from build123d import *

# Parameters (mm, degrees)
F0_R     = 35
F0_R_2   = 19
F0_R_3   = 1.5
F0_R_4   = 6.5
F0_R_5   = 3.5
F1_DEPTH = 20
F2_DEPTH = 7
F3_DEPTH = 13.75


with BuildPart() as f1:
    # F0 (on Top) → F1 (new body)
    with BuildSketch(Plane.XY):
        Circle(F0_R)
        with Locations((-7, 0)):
            Circle(F0_R_2, mode=Mode.SUBTRACT)
        with Locations((-7, 0)):
            Circle(F0_R_2)
        with Locations((-20.1270902899, -8.2419354839)):
            Circle(F0_R_3, mode=Mode.SUBTRACT)
        with Locations((-7, -15.5)):
            Circle(F0_R_3, mode=Mode.SUBTRACT)
        with Locations((6.1270902899, -8.2419354839)):
            Circle(F0_R_3, mode=Mode.SUBTRACT)
        with Locations((-20.1270902899, 8.2419354839)):
            Circle(F0_R_3, mode=Mode.SUBTRACT)
        with Locations((-7, 15.5)):
            Circle(F0_R_3, mode=Mode.SUBTRACT)
        Circle(F0_R_4, mode=Mode.SUBTRACT)
        with Locations((6.1270902899, 8.2419354839)):
            Circle(F0_R_3, mode=Mode.SUBTRACT)
        Circle(F0_R_4)
        Circle(F0_R_5, mode=Mode.SUBTRACT)
    extrude(amount=F1_DEPTH)

    # F0 (on Top) → F2 (cut)
    with BuildSketch(Plane.XY):
        with Locations((-7, 0)):
            Circle(F0_R_2)
        with Locations((-20.1270902899, -8.2419354839)):
            Circle(F0_R_3, mode=Mode.SUBTRACT)
        with Locations((-7, -15.5)):
            Circle(F0_R_3, mode=Mode.SUBTRACT)
        with Locations((6.1270902899, -8.2419354839)):
            Circle(F0_R_3, mode=Mode.SUBTRACT)
        with Locations((-20.1270902899, 8.2419354839)):
            Circle(F0_R_3, mode=Mode.SUBTRACT)
        with Locations((-7, 15.5)):
            Circle(F0_R_3, mode=Mode.SUBTRACT)
        Circle(F0_R_4, mode=Mode.SUBTRACT)
        with Locations((6.1270902899, 8.2419354839)):
            Circle(F0_R_3, mode=Mode.SUBTRACT)
    extrude(amount=F2_DEPTH, mode=Mode.SUBTRACT)

    # F3 (cut): a face of the model
    f3_faces = [f1.faces().sort_by_distance(p)[0] for p in [
        (-6.3161522369, 0, 0),
    ]]
    extrude(f3_faces, amount=-F3_DEPTH, mode=Mode.SUBTRACT)


solid = f1.part
Part model, mm, in its own coordinate system. A direction names the side the tool comes from. Round coordinates to 2 decimals unless told otherwise and drop trailing zeros. Write each loop counter-clockwise with the first axis right and the second up, starting at its lowest first coordinate (ties: lowest second). Pieces come first, ordered by that corner, then holes. Notation, with made-up numbers: M 36,5.5 L 71,5.5 A19 ccw 71,13.5 Z; hole C 61.5,-30 d4. An arc over 180 degrees is marked long. Return JSON: item names as keys, results as strings. Group by question number.
(1) Two-plate mould, pull along X, no slides. Class faces 3 (the face through (6.933, -6.977, 13.409)), 4 (the face through (15, 0, 0)), 5 (the face through (-28, -21, 10)): +X half, -X half, draft (parallel to the pull), parting line (faces both ways), or undercut.
(2) Pin check, flat tips, straight feed: pin 1 Ø2 at (x, z) = (-27.5, 11) entering from -Y; pin 2 Ø4 at (x, y) = (11, 21.5) entering from -Z; pin 3 Ø2 at (y, z) = (-24, 12.5) entering from -X; pin 4 Ø15 at (x, y) = (0, 0) entering from -Z. Stop position of each tip, or through.
(3) Which spindle directions (+Z, -Z, +X, -X, +Y, -Y) get a long thin tool onto all of the face, cutting with end or side? Do faces 1 (the face through (-25.98, 0.84, 3.45)), 2 (the face through (3.233, -1.341, 16.831)). Say none if no direction does.
(4) Saw through at B-B on x = 0. Write the cut outline in (y, z).
(5) Drill centre lines: probe 1 along Y at (x, z) = (7, 13.25); probe 2 along Y at (x, z) = (0, 11); probe 3 along Y at (x, z) = (0, 18.25). Where is each one in solid material? Low to high.
(6) Saw through at A-A on y = 0. Write the cut outline in (x, z), then the cut area to 3 significant figures.
(7) Saw through at D-D on z = 4. Write the cut outline in (x, y).
(8) Saw through at C-C on z = 11.5. Write the cut outline in (x, y).
Returned:
{
 "1": {"face 3": "undercut", "face 4": "draft", "face 5": "parting line"},
 "2": {"pin 1": "y = -22.86", "pin 2": "z = 0", "pin 3": "x = -26.38", "pin 4": "z = 7"},
 "3": {"face 1": "-Z", "face 2": "+Z, -Z"},
 "4": {"outline": "M -35,0 L -17.66,0 L -17.66,7 L -6.5,7 L -6.5,13.75 L -3.5,13.75 L -3.5,20 L -35,20 Z; M 3.5,13.75 L 6.5,13.75 L 6.5,7 L 17.66,7 L 17.66,0 L 35,0 L 35,20 L 3.5,20 Z"},
 "5": {"probe 1": "-34.29 to -9.46, -7.02 to 7.02, 9.46 to 34.29", "probe 2": "-35 to -6.5, 6.5 to 35", "probe 3": "-35 to -3.5, 3.5 to 35"},
 "6": {"outline": "M -35,0 L -26,0 L -26,7 L -6.5,7 L -6.5,13.75 L -3.5,13.75 L -3.5,20 L -35,20 Z; M 3.5,13.75 L 6.5,13.75 L 6.5,7 L 12,7 L 12,0 L 35,0 L 35,20 L 3.5,20 Z", "area": "1,000 mm²"},
 "7": {"outline": "C 0,0 d70; hole C -7,0 d38"},
 "8": {"outline": "C 0,0 d70; hole C -20.13,-8.24 d3; hole C -20.13,8.24 d3; hole C -7,-15.5 d3; hole C -7,15.5 d3; hole C 0,0 d13; hole C 6.13,-8.24 d3; hole C 6.13,8.24 d3"}
}
